Input: part model. Units: mm. Frame: model coordinates. A direction names the side the tool comes from. Round coordinates to 2 decimals unless told otherwise and drop trailing zeros. Order: outer loops, then holes, each group sorted by start corner. A loop starts at its lowest first (then second) coordinate and runs counter-clockwise, first axis right, second up. Notation, with made-up numbers: (56.5, -15) - (60.5, -15) arc R37 ccw to (60.5, 23) - close; hole circle Ø1 at (-16, -6). An arc over 180 degrees is marked (long way). One line per item, written item: value. Start each with the question number.
from build123d import *

# Parameters (mm, degrees)
F0_W     = 50
F0_H     = 30
F1_DEPTH = 14
F3_D     = 11
F5_D     = 2
F7_D     = 2
F8_R     = 5.5
F8_R_2   = 2.7
F9_DEPTH = 8


# Not quite as in the source:
# - a feature names something its author has since deleted; it is built from what else it names


with BuildPart() as f1:
    # F0 (on Top) → F1 (new body)
    with BuildSketch(Plane.XY):
        Rectangle(F0_W, F0_H)
    extrude(amount=F1_DEPTH)

    # F3 (through all)
    with Locations(Plane.XY.offset(14)):
        with Locations((0, 0)):
            Hole(F3_D / 2)

    # F5 (through all)
    with Locations(Plane.XY.offset(14)):
        with Locations((-8.9121767002, 9.0478232998), (9.0478232998, 8.9121767002), (8.9121767002, -9.0478232998), (-9.0478232998, -8.9121767002)):
            Hole(F5_D / 2)

    # F7 (through all)
    with Locations(Plane.XZ.offset(15)):
        with Locations((18, 7), (-18, 7)):
            Hole(F7_D / 2)

    # F8 (on face) → F9 (join)
    with BuildSketch(Plane.XY.offset(14)):
        Circle(F8_R)
        Circle(F8_R_2, mode=Mode.SUBTRACT)
    extrude(amount=-F9_DEPTH)


solid = f1.part
Item 1: Reachability of faces 4 (the face through (1, 3, 6)), 5 (the face through (0, -15, 7)) from +Z, -Z, +X, -X, +Y, -Y: full face, straight path, thin tool, end or side. Return the list, or none.
Item 2: First-contact query: pin 1 Ø2.5 at (x, y) = (-9.05, -8.91) entering from +Z; pin 2 Ø3.5 at (x, y) = (-1, 1) entering from -Z; pin 3 Ø1 at (x, y) = (1.5, 0) entering from -Z. Flat tips, straight axial feed; report the tip coordinate or a pass-through.
Item 3: Line query: L1, parallel to X at y = -9, z = 3.25; L2, parallel to X at y = 6.25, z = 7.25; L3, parallel to Z at x = -18, y = -5.75. Output: solid intervals per line, ascending.
Item 4: Section query D-D on x = -9. Return loops of the section in (y, z).
Item 5: Section query C-C on z = 7. Return loops of the section in (x, y), and give its area (3 significant figures).
Item 6: Pull-direction query (X, two-part tool) for faces 1 (the face through (-6, 0, 0)), 2 (the face through (25, 0, 7)), 3 (the face through (1.19, -5.37, 2.96)); classes: released by +X, released by -X, zero draft, split by the parting line, or undercut.
Item 7: Section query B-B on x = -18. Return loops of the section in (y, z), and give its area (3 significant figures).
Item 8: Section query A-A on y = 0. Return loops of the section in (x, z).
Geometry results:
1. face 4: -Z
1. face 5: +Z, -Z, +X, -X, -Y
2. pin 1: stops at z = 14
2. pin 2: stops at z = 6
2. pin 3: passes through
3. L1: x = -25 to -10.04, -8.05 to 7.91, 9.91 to 25
3. L2: x = -25 to -18.97, -17.03 to 17.03, 18.97 to 25
3. L3: z = 0 to 6, 8 to 14
4. outline: (-15, 0) - (-9.91, 0) - (-9.91, 14) - (-15, 14) - close; (-7.91, 0) - (8.05, 0) - (8.05, 14) - (-7.91, 14) - close; (10.04, 0) - (15, 0) - (15, 14) - (10.04, 14) - close
5. outline: (-25, -15) - (-19, -15) - (-19, 15) - (-25, 15) - close; (-17, -15) - (17, -15) - (17, 15) - (-17, 15) - close; (19, -15) - (25, -15) - (25, 15) - (19, 15) - close; hole circle Ø2 at (-9.05, -8.91); hole circle Ø2 at (-8.91, 9.05); hole circle Ø5.4 at (0, 0); hole circle Ø2 at (8.91, -9.05); hole circle Ø2 at (9.05, 8.91)
5. area: 1,340 mm^2
6. face 1: zero draft
6. face 2: released by +X
6. face 3: undercut
7. outline: (-15, 0) - (15, 0) - (15, 6) - (-15, 6) - close; (-15, 8) - (15, 8) - (15, 14) - (-15, 14) - close
7. area: 360 mm^2
8. outline: (-25, 0) - (-5.5, 0) - (-5.5, 6) - (-2.7, 6) - (-2.7, 14) - (-25, 14) - close; (2.7, 6) - (5.5, 6) - (5.5, 0) - (25, 0) - (25, 14) - (2.7, 14) - close; hole circle Ø2 at (-18, 7); hole circle Ø2 at (18, 7)
